The listing builds one solid part. Answer for the finished solid, in the listing's coordinates (mm). A direction names the side the tool comes from. Give positions to 0.01 mm unless a question says otherwise; leave off trailing zeros. Order: outer loops, then holes, each group sorted by start corner. A loop starts at its lowest first (then second) coordinate and runs counter-clockwise, first axis right, second up. Notation, with made-up numbers: (-8.75, 20) - (-0.75, 20) arc R22 ccw to (-0.75, 36) - close; hole circle Ø9 at (5, -34.5). An arc over 180 degrees is marked (long way). Use CSV: the item, a comma, the result in double quotes.
```python
from build123d import *

# Parameters (mm, degrees)
F0_R     = 6.604
F1_DEPTH = 12.7
F2_DEPTH = 45.72
F3_R     = 3.175
F4_DEPTH = 9.526
F5_W     = 114.3
F5_H     = 25.4
F6_DEPTH = 99.363775


with BuildPart() as f1:
    # F0 (on Front) → F1 (new body)
    with BuildSketch(Plane.XZ):
        with BuildLine():
            Line((34.847204, -35.512234), (31.675881, -29.713739))
            Line((31.675881, -29.713739), (11.365242, 7.42254))
            ThreePointArc((11.365242, 7.42254), (0, 14.160641), (-11.365242, 7.42254))
            Line((-11.365242, 7.42254), (-31.85621, -30.043455))
            Line((-31.85621, -30.043455), (-35.018866, -35.826104))
            Line((-35.018866, -35.826104), (-41.272096, -47.259603))
            Line((-41.272096, -47.259603), (-51.604832, -66.152134))
            Line((-51.604832, -66.152134), (51.604832, -66.152134))
            Line((51.604832, -66.152134), (41.11215, -46.967155))
            Line((41.11215, -46.967155), (34.847204, -35.512234))
        make_face()
        with Locations((0, 1.206641)):
            Circle(F0_R, mode=Mode.SUBTRACT)
    extrude(amount=F1_DEPTH)

    # F0 (on Front) → F2 (join)
    with BuildSketch(Plane.XZ):
        Polygon((63.5, -66.152134), (51.604832, -66.152134), (-51.604832, -66.152134), (-63.5, -66.152134), (-63.5, -75.677134), (-88.9, -75.677134), (-88.9, -85.202134), (88.9, -85.202134), (88.9, -75.677134), (63.5, -75.677134), align=None)
    extrude(amount=F2_DEPTH)

    # F3 (on face) → F4 (cut, through all)
    with BuildSketch(Plane.XY.offset(-75.677134)):
        with Locations((-76.302797, -12.066366)):
            Circle(F3_R)
        with Locations((-76.302797, -33.448037)):
            Circle(F3_R)
        with Locations((76.302797, -12.066366)):
            Circle(F3_R)
        with Locations((76.302797, -33.448037)):
            Circle(F3_R)
    extrude(amount=-F4_DEPTH, mode=Mode.SUBTRACT)

    # F5 (on face) → F6 (cut, through all)
    with BuildSketch(Plane(origin=(0, 0, -85.202134), x_dir=(1, 0, 0), z_dir=(0, 0, -1))):
        with Locations((0, 33.02)):
            Rectangle(F5_W, F5_H)
    extrude(amount=-F6_DEPTH, mode=Mode.SUBTRACT)


solid = f1.part
```
Item 1: Each of these flat-tipped pins is pushed along its axis until it touches: pin 1 (24 mm diameter, centred on x = -4, z = -41.5, fed in from -Y); pin 2 (8.5 mm diameter, centred on x = -76.3, y = -33.45, fed in from -Z); pin 3 (7.5 mm diameter, centred on x = 81, y = -18, fed in from +Z); pin 4 (1 mm diameter, centred on y = -9.5, z = -0.5, fed in from +X). Where does it stop, or does it pass through?
Taken from the geometry:
pin 1,"y = -12.7"
pin 2,"z = -85.2"
pin 3,"z = -75.68"
pin 4,"x = 15.97"
Item 2: Find the intervals of material crossed by line 1 along Z through (x, y) = (38, -13.5); line 2 along Z through (x, y) = (-80, -30); line 3 along Y through (x, z) = (-42.5, -64), in increasing order.
Taken from the geometry:
line 1,"-85.2 to -66.15"
line 2,"-85.2 to -75.68"
line 3,"-12.7 to 0"
Item 3: Which of the six approach directions +Z, -Z, +X, -X, +Y, -Y give full straight-line access (tool end or side, diameter ignored) to faces 5 (the face through (-1, -12.7, -34)), 6 (the face through (63.5, -23, -71)), 7 (the face through (-63.5, -23, -71)), 8 (the face through (57.15, -33, -76)), 9 (the face through (-79.475, -11.927, -80.373))?
Taken from the geometry:
face 5,"+Z, +X, -X, -Y"
face 6,"+Z, +X, +Y, -Y"
face 7,"+Z, -X, +Y, -Y"
face 8,"+Z, -Z, -Y"
face 9,"+Z, -Z"
Item 4: The part is cut by section A-A (x = 0). Give the vertices of the cut face in (y, z), and give its area (3 significant figures).
Taken from the geometry:
outline,"(-20.32, -85.2) - (0, -85.2) - (0, -5.4) - (-12.7, -5.4) - (-12.7, -66.15) - (-20.32, -66.15) - close; (-12.7, 7.81) - (0, 7.81) - (0, 14.16) - (-12.7, 14.16) - close"
area,"1,240 mm^2"
Item 5: The part is cut by section C-C (z = -73). Give the vertices of the cut face in (x, y).
Taken from the geometry:
outline,"(-63.5, -45.72) - (-57.15, -45.72) - (-57.15, -20.32) - (57.15, -20.32) - (57.15, -45.72) - (63.5, -45.72) - (63.5, 0) - (-63.5, 0) - close"
Item 6: The mould has two halves that part along Y. Classify faces 1 (the face through (73.13, -11.93, -80.37)), 2 (the face through (-1.43, -6.26, -5.24)), 3 (the face through (-78.82, -35.38, -80.37)), 4 (the face through (-70, -45.72, -80)): +Y half, -Y half, draft (parallel to the pull), parting line (faces both ways), or undercut.
Taken from the geometry:
face 1,"undercut"
face 2,"draft"
face 3,"undercut"
face 4,"-Y half"
Item 7: The part is cut by section D-D (y = -6). Give the vertices of the cut face in (x, z).
Taken from the geometry:
outline,"(-88.9, -85.2) - (88.9, -85.2) - (88.9, -75.68) - (63.5, -75.68) - (63.5, -66.15) - (51.6, -66.15) - (11.37, 7.42) arc R12.95 ccw to (-11.37, 7.42) - (-51.6, -66.15) - (-63.5, -66.15) - (-63.5, -75.68) - (-88.9, -75.68) - close; hole circle Ø13.21 at (0, 1.21)"
Item 8: The part is cut by section B-B (y = -26). Give the vertices of the cut face in (x, z), and give its area (3 significant figures).
Taken from the geometry:
outline,"(-88.9, -85.2) - (-57.15, -85.2) - (-57.15, -66.15) - (-63.5, -66.15) - (-63.5, -75.68) - (-88.9, -75.68) - close; (57.15, -85.2) - (88.9, -85.2) - (88.9, -75.68) - (63.5, -75.68) - (63.5, -66.15) - (57.15, -66.15) - close"
area,"726 mm^2"
